Check sheet for the modelled part. Datum: model origin and axes. Units: mm. A direction names the side the tool comes from. Round coordinates to 2 decimals unless told otherwise and drop trailing zeros. Write each loop counter-clockwise with the first axis right and the second up, starting at its lowest first coordinate (ties: lowest second). Pieces come first, ordered by that corner, then holes. Notation, with made-up numbers: M 16,30.25 L 42,30.25 A11 cw 42,42.25 Z; hole C 46,66 d2. An arc over 180 degrees is marked long. Put each result on its own line as item: value.
```python
from build123d import *

# Parameters (mm, degrees)
SKETCH1_W           = 53
SKETCH1_H           = 32.5
BOSS_EXTRUDE1_DEPTH = 3
SKETCH5_W           = 6
SKETCH5_H           = 3
BOSS_EXTRUDE2_DEPTH = 20
SKETCH6_R           = 2.15
CUT_EXTRUDE3_DEPTH  = 10
SKETCH7_W           = 2.4
SKETCH7_H           = 5.5
CUT_EXTRUDE6_DEPTH  = 10
SKETCH8_R           = 1.5
CUT_EXTRUDE7_DEPTH  = 10
BOSS_EXTRUDE3_DEPTH = 6
BOSS_EXTRUDE4_DEPTH = 6


with BuildPart() as part:
    # Sketch1 → Boss-Extrude1 (new body)
    with BuildSketch(Plane.XY):
        with Locations((9.74034322, 3.310344828)):
            Rectangle(SKETCH1_W, SKETCH1_H)
    extrude(amount=BOSS_EXTRUDE1_DEPTH)

    # Sketch5 → Boss-Extrude2 (add)
    with BuildSketch(Plane(origin=(0, 0, 0), x_dir=(-1, 0, 0), z_dir=(0, 0, -1))):
        with Locations((-33.24034322, 12.060344828)):
            Rectangle(SKETCH5_W, SKETCH5_H)
        with Locations((13.75965678, 12.060344828)):
            Rectangle(SKETCH5_W, SKETCH5_H)
    extrude(amount=BOSS_EXTRUDE2_DEPTH)

    # Sketch6 → Cut-Extrude3 (cut)
    with BuildSketch(Plane(origin=(0, 13.560344828, 0), x_dir=(1, 0, 0), z_dir=(0, 1, 0))):
        with Locations(Location((33.64034322, 4.9, 0), (0, 0, 270))):
            Circle(SKETCH6_R)
        with Locations(Location((33.64034322, 15.1, 0), (0, 0, 270))):
            Circle(SKETCH6_R)
        with Locations(Location((-14.15965678, 4.9, 0), (0, 0, 270))):
            Circle(SKETCH6_R)
        with Locations(Location((-14.15965678, 15.1, 0), (0, 0, 270))):
            Circle(SKETCH6_R)
    extrude(amount=-CUT_EXTRUDE3_DEPTH, mode=Mode.SUBTRACT)

    # Sketch7 → Cut-Extrude6 (cut)
    with BuildSketch(Plane(origin=(0, 0, 0), x_dir=(-1, 0, 0), z_dir=(0, 0, -1))):
        with Locations((8.172781941, 11.783549127)):
            Rectangle(SKETCH7_W, SKETCH7_H)
    extrude(amount=-CUT_EXTRUDE6_DEPTH, mode=Mode.SUBTRACT)

    # Sketch8 → Cut-Extrude7 (cut)
    with BuildSketch(Plane(origin=(0, 0, 0), x_dir=(-1, 0, 0), z_dir=(0, 0, -1))):
        with Locations((-33.24034322, 4.560344828)):
            Circle(SKETCH8_R)
        with Locations((-33.24034322, -8.439655172)):
            Circle(SKETCH8_R)
        with Locations((13.75965678, -8.439655172)):
            Circle(SKETCH8_R)
        with Locations((13.75965678, 4.560344828)):
            Circle(SKETCH8_R)
    extrude(amount=-CUT_EXTRUDE7_DEPTH, mode=Mode.SUBTRACT)

    # Sketch9 → Boss-Extrude3 (add)
    with BuildSketch(Plane.ZY.offset(16.75965678)):
        Polygon((-2, 10.560344828), (0, 10.560344828), (0, 7.560344828), align=None)
    extrude(amount=-BOSS_EXTRUDE3_DEPTH)

    # Sketch10 → Boss-Extrude4 (add)
    with BuildSketch(Plane(origin=(36.24034322, 0, 0), x_dir=(0, 0, -1), z_dir=(1, 0, 0))):
        Polygon((2, 10.560344828), (0, 10.560344828), (0, 7.560344828), align=None)
    extrude(amount=-BOSS_EXTRUDE4_DEPTH)


solid = part.part
```
1. Depth check by flat-ended pin: pin 1 Ø1.8 at (x, z) = (-15, -13) entering from -Y; pin 2 Ø1.8 at (x, y) = (33.24, -8.44) entering from -Z; pin 3 Ø7 at (x, z) = (-14.16, -4.9) entering from +Y; pin 4 Ø8 at (x, y) = (25, -5.5) entering from -Z. Enter the tip coordinate at first touch or a pass-through.
Computed values:
pin 1: stops at y = 10.56
pin 2: passes through
pin 3: stops at y = 13.56
pin 4: stops at z = 0
2. Cross-section at D-D (z = -16.25). Enter the section's corners in (x, y).
Computed values:
outline: M -16.76,10.56 L -15.98,10.56 L -15.98,13.56 L -16.76,13.56 Z; M -12.34,10.56 L -10.76,10.56 L -10.76,13.56 L -12.34,13.56 Z; M 30.24,10.56 L 31.82,10.56 L 31.82,13.56 L 30.24,13.56 Z; M 35.46,10.56 L 36.24,10.56 L 36.24,13.56 L 35.46,13.56 Z
3. Cross-section at B-B (z = -4.9). Enter the section's corners in (x, y).
Computed values:
outline: M -16.76,10.56 L -16.31,10.56 L -16.31,13.56 L -16.76,13.56 Z; M -12.01,10.56 L -10.76,10.56 L -10.76,13.56 L -12.01,13.56 Z; M 30.24,10.56 L 31.49,10.56 L 31.49,13.56 L 30.24,13.56 Z; M 35.79,10.56 L 36.24,10.56 L 36.24,13.56 L 35.79,13.56 Z
4. Cross-section at C-C (y = 10). Enter the section's corners in (x, z).
Computed values:
outline: M -16.76,-1.63 L -10.76,-1.63 L -10.76,0 L -9.37,0 L -9.37,3 L -16.76,3 Z; M -6.97,0 L 30.24,0 L 30.24,-1.63 L 36.24,-1.63 L 36.24,3 L -6.97,3 Z
5. Cross-section at A-A (x = -8.5). Enter the section's corners in (y, z).
Computed values:
outline: M -12.94,0 L 9.03,0 L 9.03,3 L -12.94,3 Z; M 14.53,0 L 19.56,0 L 19.56,3 L 14.53,3 Z
6. Scan lines: probe 1 along X at (y, z) = (12.4, -4.9); probe 2 along Y at (x, z) = (33, -18.25); probe 3 along Z at (x, y) = (27.5, 18). Record each from-to range of solid material in increasing order.
Computed values:
probe 1: x = -16.76 to -16.31, -12.01 to -10.76, 30.24 to 31.49, 35.79 to 36.24
probe 2: y = 10.56 to 13.56
probe 3: z = 0 to 3
7. Access from +Z, -Z, +X, -X, +Y, -Y to the whole of each face (thin tool, end or side, straight path). Record for faces 1 (the flat face through (-14, 12, -20)), 2 (the flat face through (-8, 14.534, 1)), 3 (the flat face through (30.24, 12, -10)), 4 (the flat face through (33, 10.56, -11)), 5 (the cylindrical face through (35.093, 12.081, -6.485)).
Computed values:
face 1: -Z, +X, -X, +Y, -Y
face 2: +Z, -Z
face 3: -Z, +Y, -Y
face 4: -Z, +X, -X, -Y
face 5: +Y, -Y
8. Release check for a two-part mould opening along X. For faces 6 (the cylindrical face through (31.855, 3.986, 1.479)), 7 (the flat face through (33, 12, -20)) record: +X half, -X half, draft (parallel to the pull), parting line (faces both ways), or undercut.
Computed values:
face 6: undercut
face 7: draft
